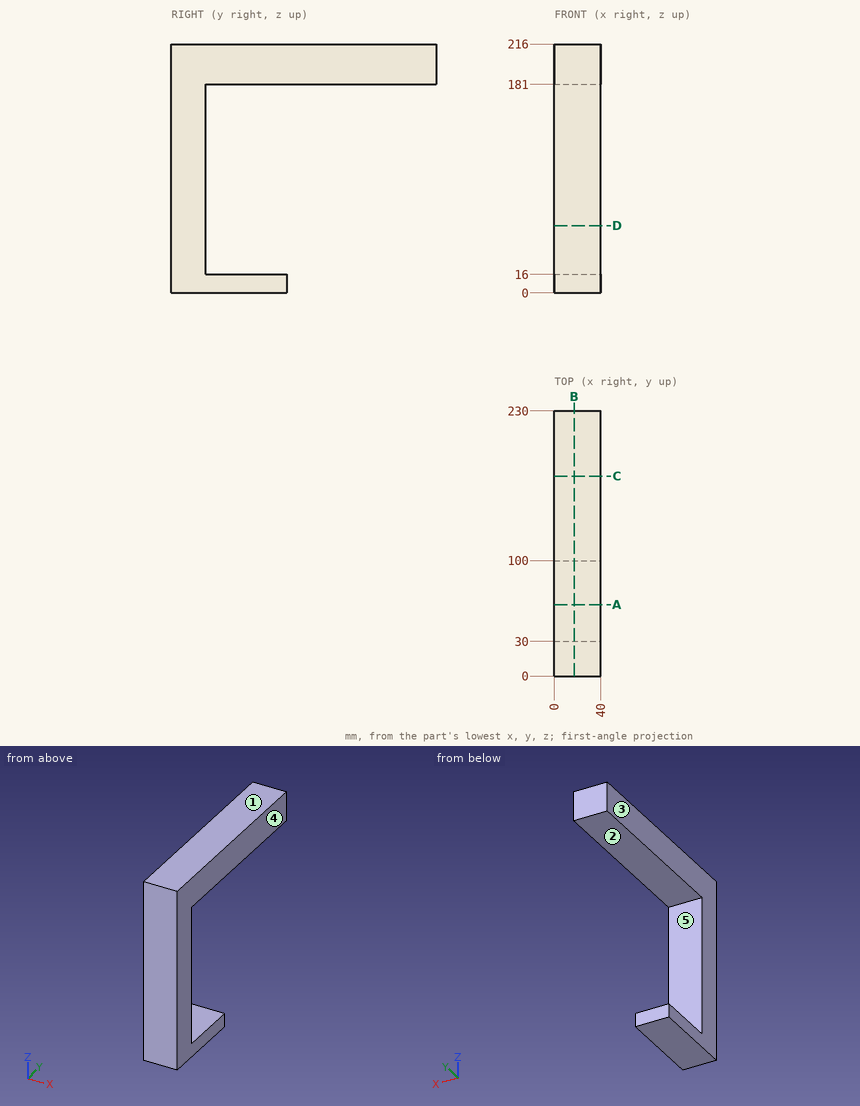
Job drawing, mm, ordinate dimensions from the low corner. One solid piece. A direction names the side the tool comes from. Give positions to 0.01 mm unless a question says otherwise; leave off trailing zeros. Loops run counter-clockwise (first coordinate to the right, second up) from the corner with the lowest first, then second, coordinate; pieces in that order, holes last. Notation, with made-up numbers: (35, 48.5) -> (41, 48.5) arc R22 ccw to (41, 66.5) -> close; hole circle Ø11 at (-21.75, -22). An arc over 180 degrees is marked (long way). Use a Markdown table: item, result. Add a question column.
(1) Wall check: line 1 along Z through (x, y) = (36, 64); line 2 along Z through (x, y) = (22.5, 141.5); line 3 along Y through (x, z) = (12.5, 77.5). Give the ranges that are in metal, low to high.
(2) Slice it at D-D on z = 58.5. List the corners of the cut face in (x, y), and give its area (3 significant figures).
(3) Slice it at C-C on y = 173.5. List the corners of the cut face in (x, z), and give its area (3 significant figures).
(4) Drop flat-ended pins along their axis: pin 1 Ø1.5 at (x, z) = (34, 29) entering from +Y; pin 2 Ø20 at (x, y) = (16.5, 168.5) entering from -Z; pin 3 Ø13 at (x, z) = (18, 9) entering from +Y. Give the stop position or say it passes through.
(5) Slice it at B-B on x = 17. List the corners of the cut face in (y, z).
(6) Slice it at A-A on y = 62. List the corners of the cut face in (x, z), and give its area (3 significant figures).
(7) Mould opens along Z. For the marked faces 1, 2 and 3 say: +Z half, -Z half, draft (parallel to the pull), parting line (faces both ways), or undercut.
(8) Tool access for the marked faces 4 and 5: list every direction of +Z, -Z, +X, -X, +Y, -Y with a clear straight run to the whole face (end or side of a thin tool).
Filled sheet:
| question | item | result |
|---|---|---|
| 1 | line 1 | 0 to 16, 181 to 216 |
| 1 | line 2 | 181 to 216 |
| 1 | line 3 | 0 to 30 |
| 2 | outline | (0, 0) -> (40, 0) -> (40, 30) -> (0, 30) -> close |
| 2 | area | 1,200 mm2 |
| 3 | outline | (0, 181) -> (40, 181) -> (40, 216) -> (0, 216) -> close |
| 3 | area | 1,400 mm2 |
| 4 | pin 1 | y = 30 |
| 4 | pin 2 | z = 181 |
| 4 | pin 3 | y = 100 |
| 5 | outline | (0, 0) -> (100, 0) -> (100, 16) -> (30, 16) -> (30, 181) -> (230, 181) -> (230, 216) -> (0, 216) -> close |
| 6 | outline | (0, 0) -> (40, 0) -> (40, 16) -> (0, 16) -> close; (0, 181) -> (40, 181) -> (40, 216) -> (0, 216) -> close |
| 6 | area | 2,040 mm2 |
| 7 | face 1 | +Z half |
| 7 | face 2 | undercut |
| 7 | face 3 | draft |
| 8 | face 4 | +Z, -Z, +X, +Y, -Y |
| 8 | face 5 | +X, -X, +Y |
